Input: part model. Units: mm. Frame: model coordinates. Face numbers are marked on the shaded views. A direction names the side the tool comes from. Coordinates: 2 decimals unless noted, no trailing zeros. Order: outer loops, then holes, each group sorted by start corner. A loop starts at its lowest first (then second) coordinate and runs counter-clockwise, first axis right, second up. Notation, with made-up numbers: (62.5, -17.5) - (119.5, -17.5) arc R29 cw to (119.5, 19.5) - close; hole circle Ø4 at (-12, 14.25). An arc over 180 degrees is marked (long way). One line per question, with ' | ' between items.
from build123d import *

# Parameters (mm, degrees)
SKETCH1_W                        = 200
SKETCH1_H                        = 60
BOSS_EXTRUDE1_DEPTH              = 20
SKETCH2_W                        = 150
SKETCH2_H                        = 60
CUT_EXTRUDE1_DEPTH               = 5
SKETCH5_R                        = 7
BOSS_EXTRUDE2_DEPTH              = 15
RIB1_START                       = -5
RIB1_DEPTH                       = 10
SKETCH7_R                        = 16.25
SKETCH7_R_2                      = 7
BOSS_EXTRUDE3_DEPTH              = 4
FILLET1_R                        = 10
FILLET2_R                        = 2
F_10_0MM_DOWEL_HOLE2_D           = 10
F_10_0MM_DOWEL_HOLE2_CSINK_D     = 10.05
F_10_0MM_DOWEL_HOLE2_CSINK_ANGLE = 90


# Read off the part's stored shape, not the designer's step: Rib1
with BuildPart() as part:
    # Sketch1 → Boss-Extrude1 (new body)
    with BuildSketch(Plane(origin=(0, 0, 0), x_dir=(1, 0, 0), z_dir=(0, 1, 0))):
        Rectangle(SKETCH1_W, SKETCH1_H)
    extrude(amount=BOSS_EXTRUDE1_DEPTH)

    # Sketch2 → Cut-Extrude1 (cut)
    with BuildSketch(Plane(origin=(0, 20, 0), x_dir=(1, 0, 0), z_dir=(0, 1, 0))):
        Rectangle(SKETCH2_W, SKETCH2_H)
    extrude(amount=-CUT_EXTRUDE1_DEPTH, mode=Mode.SUBTRACT)

    # Sketch5 → Boss-Extrude2 (add)
    with BuildSketch(Plane(origin=(-32.5, 0, 0), x_dir=(0, 0, -1), z_dir=(1, 0, 0))):
        with BuildLine():
            Line((-30, 15), (-30, 50))
            ThreePointArc((-30, 50), (0, 80), (30, 50))
            Line((30, 50), (30, 15))
            Line((30, 15), (-30, 15))
        make_face()
        with Locations((0, 50)):
            Circle(SKETCH5_R, mode=Mode.SUBTRACT)
    boss_extrude2 = extrude(amount=BOSS_EXTRUDE2_DEPTH)

    # Rib1 outline → Rib1 (add)
    with BuildSketch(Plane.XY.offset(RIB1_START)):
        Polygon((-37.5, 40), (-75, 20), (-75, 15), (-32.5, 15), (-32.5, 40), align=None)
    rib1 = extrude(amount=RIB1_DEPTH)

    # Sketch7 → Boss-Extrude3 (add)
    with BuildSketch(Plane(origin=(-17.5, 0, 0), x_dir=(0, 0, -1), z_dir=(1, 0, 0))):
        with Locations(Location((0, 50, 0), (0, 0, 180))):
            Circle(SKETCH7_R)
        with Locations((0, 50)):
            Circle(SKETCH7_R_2, mode=Mode.SUBTRACT)
    boss_extrude3 = extrude(amount=BOSS_EXTRUDE3_DEPTH)

    # Mirror1: Boss-Extrude2, Rib1, Boss-Extrude3 across plane
    add(boss_extrude2.mirror(Plane(origin=(0, 0, 0), x_dir=(0, 0, 1), z_dir=(1, 0, 0))))
    add(rib1.mirror(Plane(origin=(0, 0, 0), x_dir=(0, 0, 1), z_dir=(1, 0, 0))))
    add(boss_extrude3.mirror(Plane(origin=(0, 0, 0), x_dir=(0, 0, 1), z_dir=(1, 0, 0))))

    # Fillet1
    fillet1_edges = [part.edges().sort_by_distance(p)[0] for p in [
        (100, 10, 30),
        (-100, 10, 30),
        (-100, 10, -30),
        (100, 10, -30),
    ]]
    fillet(fillet1_edges, radius=FILLET1_R)

    # Fillet2
    fillet2_edges = [part.edges().sort_by_distance(p)[0] for p in [
        (32.5, 15, -17.5),
        (75, 15, -17.5),
        (17.5, 50, -16.25),
        (75, 15, 17.5),
        (-75, 15, -17.5),
        (-17.5, 15, 0),
        (-32.5, 15, 17.5),
        (-32.5, 15, -17.5),
        (-75, 15, 17.5),
        (-17.5, 50, -16.25),
        (17.5, 15, 0),
        (32.5, 15, 17.5),
    ]]
    fillet(fillet2_edges, radius=FILLET2_R)

    # Ø10.0mm Dowel Hole2 (through all)
    with Locations(Plane(origin=(0, 20, 0), x_dir=(1, 0, 0), z_dir=(0, 1, 0))):
        with Locations((-87.631640785, 16.25), (-87.345692882, -16.25), (87.368359215, 16.25), (87.781361724, -16.247375724)):
            CounterSinkHole(F_10_0MM_DOWEL_HOLE2_D / 2, F_10_0MM_DOWEL_HOLE2_CSINK_D / 2, counter_sink_angle=F_10_0MM_DOWEL_HOLE2_CSINK_ANGLE)


solid = part.part
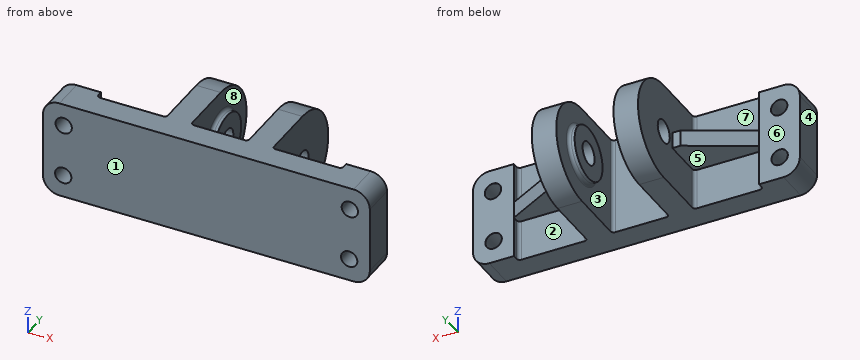
Item 1: Access query for the marked faces 5, 6, 7 and 8. Directions: +Z, -Z, +X, -X, +Y, -Y. A direction counts if a zero-diameter tool reaches every point of the face in a straight line with its end or side. Return the directions, or none.
Data:
face 5: -Z, +Y | face 6: +Z, -Z, -X, +Y | face 7: +Z, +Y | face 8: none
Item 2: Section A-A on x = 26. Return the cut outline in (y, z).
Data:
outline: (0, -30) - (50, -30) arc R30 ccw to (50, 30) - (0, 30) - close; hole circle Ø14 at (50, 0)
Item 3: Ray query, line 1 (X direction, y = 38, z = -6); line 2 (X direction, y = 32, z = -25); line 3 (X direction, y = 10, z = 16). Return the intervals inside material, ascending.
Data:
line 1: -32.5 to -13.5, 13.5 to 32.5 | line 2: -32.5 to -17.5, 17.5 to 32.5 | line 3: -100 to -92.34, -82.35 to 82.79, 92.78 to 100
Item 4: Section B-B on z = 0. Count the separate pieces of the cut face and the enclosed holes in it, and give its area (3 significant figures).
Data:
separate pieces: 3 | enclosed holes: 0 | area: 6,310 mm^2
Item 5: Contact query for flat-ended pins moving along their axis: P1, Ø1, axis at y = 71.5, z = -12, coming from the -X side; P2, Ø3, axis at x = -21.5, y = 56, coming from the +Z side; P3, Ø9.5, axis at x = 6, z = 4, coming from the +Y side; P4, Ø20, axis at x = 48.5, y = 24.5, coming from the +Z side. Output: stop coordinate, or through.
Data:
P1: x = -32.5 | P2: z = 29.66 | P3: y = 15 | P4: z = 30
Item 6: Section D-D on z = 24. Return the cut outline in (x, y), and give its area (3 significant figures).
Data:
outline: (-99.17, 0) - (99.17, 0) - (99.17, 20) - (75, 20) - (75, 17) arc R2 cw to (73, 15) - (34.5, 15) arc R2 cw to (32.5, 17) - (32.5, 68) - (17.5, 68) - (17.5, 17) arc R2 cw to (15.5, 15) - (-15.5, 15) arc R2 cw to (-17.5, 17) - (-17.5, 68) - (-32.5, 68) - (-32.5, 17) arc R2 cw to (-34.5, 15) - (-73, 15) arc R2 cw to (-75, 17) - (-75, 20) - (-99.17, 20) - close | area: 4,810 mm^2
Item 7: Draft query along Y for the marked faces 1, 2, 3 and 4. Return one class per face: released by +Y, released by -Y, zero draft, split by the parting line, or undercut.
Data:
face 1: released by -Y | face 2: released by +Y | face 3: undercut | face 4: zero draft
Item 8: Section C-C on y = 10. Return the cut outline in (x, z).
Data:
outline: (-100, -20) arc R10 ccw to (-90, -30) - (90, -30) arc R10 ccw to (100, -20) - (100, 20) arc R10 ccw to (90, 30) - (-90, 30) arc R10 ccw to (-100, 20) - close; hole circle Ø10 at (-87.63, -16.25); hole circle Ø10 at (-87.35, 16.25); hole circle Ø10 at (87.37, -16.25); hole circle Ø10 at (87.78, 16.25)
